```python
from build123d import *

# Parameters (mm, degrees)
F0_R     = 2.0955
F2_DEPTH = 500


with BuildPart() as f2:
    # F0 (on Front) → F2 (new body)
    with BuildSketch(Plane.XZ):
        with BuildLine():
            Line((-4.6246692655, 9.9949), (-9.0043, 9.9949))
            ThreePointArc((-9.0043, 9.9949), (-9.7047599774, 9.7047599774), (-9.9949, 9.0043))
            Line((-9.9949, 9.0043), (-9.9949, 4.6246692655))
            Line((-9.9949, 4.6246692655), (-8.1915, 2.8212692655))
            Line((-8.1915, 2.8212692655), (-8.1915, 5.4628692655))
            Line((-8.1915, 5.4628692655), (-6.5405, 5.4628692655))
            Line((-6.5405, 5.4628692655), (-3.8989, 2.8212692655))
            Line((-3.8989, 2.8212692655), (-3.8989, -2.8212692655))
            Line((-3.8989, -2.8212692655), (-6.5405, -5.4628692655))
            Line((-6.5405, -5.4628692655), (-8.1915, -5.4628692655))
            Line((-8.1915, -5.4628692655), (-8.1915, -2.8212692655))
            Line((-8.1915, -2.8212692655), (-9.9949, -4.6246692655))
            Line((-9.9949, -4.6246692655), (-9.9949, -9.0043))
            ThreePointArc((-9.9949, -9.0043), (-9.7047599774, -9.7047599774), (-9.0043, -9.9949))
            Line((-9.0043, -9.9949), (-4.6246692655, -9.9949))
            Line((-4.6246692655, -9.9949), (-2.8212692655, -8.1915))
            Line((-2.8212692655, -8.1915), (-5.4628692655, -8.1915))
            Line((-5.4628692655, -8.1915), (-5.4628692655, -6.5405))
            Line((-5.4628692655, -6.5405), (-2.8212692655, -3.8989))
            Line((-2.8212692655, -3.8989), (2.8212692655, -3.8989))
            Line((2.8212692655, -3.8989), (5.4628692655, -6.5405))
            Line((5.4628692655, -6.5405), (5.4628692655, -8.1915))
            Line((5.4628692655, -8.1915), (2.8212692655, -8.1915))
            Line((2.8212692655, -8.1915), (4.6246692655, -9.9949))
            Line((4.6246692655, -9.9949), (9.0043, -9.9949))
            ThreePointArc((9.0043, -9.9949), (9.7047599774, -9.7047599774), (9.9949, -9.0043))
            Line((9.9949, -9.0043), (9.9949, -4.6246692655))
            Line((9.9949, -4.6246692655), (8.1915, -2.8212692655))
            Line((8.1915, -2.8212692655), (8.1915, -5.4628692655))
            Line((8.1915, -5.4628692655), (6.5405, -5.4628692655))
            Line((6.5405, -5.4628692655), (3.8989, -2.8212692655))
            Line((3.8989, -2.8212692655), (3.8989, 2.8212692655))
            Line((3.8989, 2.8212692655), (6.5405, 5.4628692655))
            Line((6.5405, 5.4628692655), (8.1915, 5.4628692655))
            Line((8.1915, 5.4628692655), (8.1915, 2.8212692655))
            Line((8.1915, 2.8212692655), (9.9949, 4.6246692655))
            Line((9.9949, 4.6246692655), (9.9949, 9.0043))
            ThreePointArc((9.9949, 9.0043), (9.7047599774, 9.7047599774), (9.0043, 9.9949))
            Line((9.0043, 9.9949), (4.6246692655, 9.9949))
            Line((4.6246692655, 9.9949), (2.8212692655, 8.1915))
            Line((2.8212692655, 8.1915), (5.4628692655, 8.1915))
            Line((5.4628692655, 8.1915), (5.4628692655, 6.5405))
            Line((5.4628692655, 6.5405), (2.8212692655, 3.8989))
            Line((2.8212692655, 3.8989), (-2.8212692655, 3.8989))
            Line((-2.8212692655, 3.8989), (-5.4628692655, 6.5405))
            Line((-5.4628692655, 6.5405), (-5.4628692655, 8.1915))
            Line((-5.4628692655, 8.1915), (-2.8212692655, 8.1915))
            Line((-2.8212692655, 8.1915), (-4.6246692655, 9.9949))
        make_face()
        with BuildLine():
            ThreePointArc((-8.0391, -8.1915), (-8.1468630735, -8.1468630735), (-8.1915, -8.0391))
            Line((-8.1915, -8.0391), (-8.1915, -6.6929))
            ThreePointArc((-8.1915, -6.6929), (-8.1468630735, -6.5851369265), (-8.0391, -6.5405))
            Line((-8.0391, -6.5405), (-7.9883, -6.5405))
            Line((-7.9883, -6.5405), (-6.5405, -7.9883))
            Line((-6.5405, -7.9883), (-6.5405, -8.0391))
            ThreePointArc((-6.5405, -8.0391), (-6.5851369265, -8.1468630735), (-6.6929, -8.1915))
            Line((-6.6929, -8.1915), (-8.0391, -8.1915))
        make_face(mode=Mode.SUBTRACT)
        with BuildLine():
            Line((8.1915, -6.6929), (8.1915, -8.0391))
            ThreePointArc((8.1915, -8.0391), (8.1468630735, -8.1468630735), (8.0391, -8.1915))
            Line((8.0391, -8.1915), (6.6929, -8.1915))
            ThreePointArc((6.6929, -8.1915), (6.5851369265, -8.1468630735), (6.5405, -8.0391))
            Line((6.5405, -8.0391), (6.5405, -7.9883))
            Line((6.5405, -7.9883), (7.9883, -6.5405))
            Line((7.9883, -6.5405), (8.0391, -6.5405))
            ThreePointArc((8.0391, -6.5405), (8.1468630735, -6.5851369265), (8.1915, -6.6929))
        make_face(mode=Mode.SUBTRACT)
        with BuildLine():
            Line((-7.9883, 6.5405), (-8.0391, 6.5405))
            ThreePointArc((-8.0391, 6.5405), (-8.1468630735, 6.5851369265), (-8.1915, 6.6929))
            Line((-8.1915, 6.6929), (-8.1915, 8.0391))
            ThreePointArc((-8.1915, 8.0391), (-8.1468630735, 8.1468630735), (-8.0391, 8.1915))
            Line((-8.0391, 8.1915), (-6.6929, 8.1915))
            ThreePointArc((-6.6929, 8.1915), (-6.5851369265, 8.1468630735), (-6.5405, 8.0391))
            Line((-6.5405, 8.0391), (-6.5405, 7.9883))
            Line((-6.5405, 7.9883), (-7.9883, 6.5405))
        make_face(mode=Mode.SUBTRACT)
        Circle(F0_R, mode=Mode.SUBTRACT)
        with BuildLine():
            ThreePointArc((8.1915, 6.6929), (8.1468630735, 6.5851369265), (8.0391, 6.5405))
            Line((8.0391, 6.5405), (7.9883, 6.5405))
            Line((7.9883, 6.5405), (6.5405, 7.9883))
            Line((6.5405, 7.9883), (6.5405, 8.0391))
            ThreePointArc((6.5405, 8.0391), (6.5851369265, 8.1468630735), (6.6929, 8.1915))
            Line((6.6929, 8.1915), (8.0391, 8.1915))
            ThreePointArc((8.0391, 8.1915), (8.1468630735, 8.1468630735), (8.1915, 8.0391))
            Line((8.1915, 8.0391), (8.1915, 6.6929))
        make_face(mode=Mode.SUBTRACT)
    extrude(amount=F2_DEPTH)


solid = f2.part
```
Source: CAD feature listing. Evaluate the final solid. Frame: model axes, mm. Round coordinates to 2 decimals unless told otherwise and drop trailing zeros. Answer as a JSON object with one key per item and string values. Group by question number.
(1) First-contact query: pin 1 (6 mm diameter, centred on y = -349, z = -1.5, fed in from +X); pin 2 (4 mm diameter, centred on x = 0, z = 0, fed in from +Y); pin 3 (3 mm diameter, centred on y = -167, z = 0.5, fed in from -X); pin 4 (2 mm diameter, centred on x = 2, y = -326, fed in from -Z). Flat tips, straight axial feed; report the tip coordinate or a pass-through.
(2) Section query A-A on y = -462.5. State how many separate pieces and enclosed holes the cut face has, then the cut area to 3 significant figures.
(3) Ray query, line 1 (Z direction, x = -8, y = -364); line 2 (X direction, y = -236, z = -6.5). Return the intervals inside material, ascending. Write a range as [from, to].
Computed values:
{
 "1": {"pin 1": "x = 9.87", "pin 2": "through", "pin 3": "x = -3.9", "pin 4": "z = -8.37"},
 "2": {"separate pieces": "1", "enclosed holes": "5", "area": "165 mm^2"},
 "3": {"line 1": "[-9.99, -8.19], [-6.54, -5.46], [5.46, 6.54], [8.19, 9.99]", "line 2": "[-9.99, -5.42], [5.42, 9.99]"}
}
